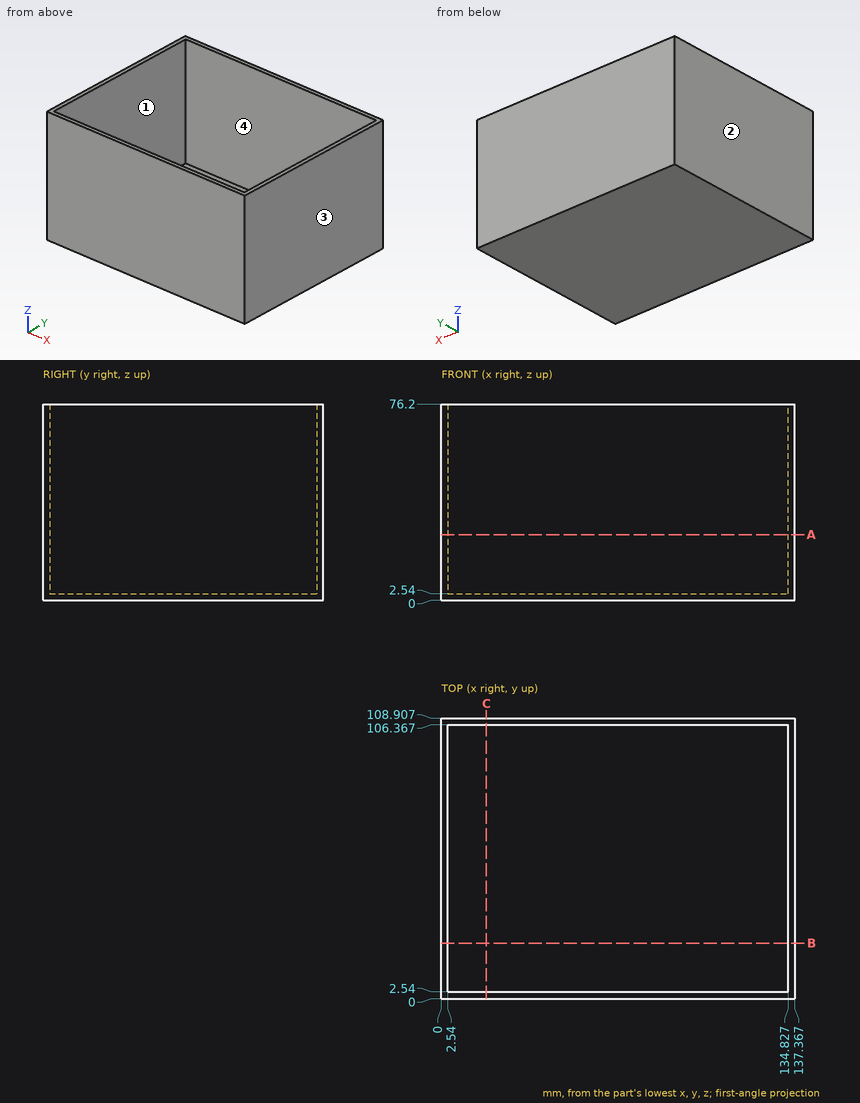
Input: dimensioned drawing with shaded views. Units: mm. Origin: part minimum x, y, z. Coordinates: 2 decimals unless noted, no trailing zeros. Loops run counter-clockwise (first coordinate to the right, second up) from the corner with the lowest first, then second, coordinate; pieces in that order, holes last. Notation, with made-up numbers: (-24.5, 37) - (27.5, 37) arc R15 ccw to (27.5, 66) - close; hole circle Ø9 at (74.25, 23.5). An arc over 180 degrees is marked (long way). One line per question, with ' | ' between items. Start each with the question number.
(1) Cut plane C-C on x = 17.5. Output: boundary loops of the cut face in (y, z).
(2) Ray query, L1, parallel to Y at x = 63.5, z = 60.5; L2, parallel to X at y = 36.5, z = 43; L3, parallel to Z at x = 30, y = 92.5. Return the intervals inside material, ascending. Write a range as from..to.
(3) Cut plane B-B on y = 21.5. Output: boundary loops of the cut face in (x, z).
(4) Draft query along X for the marked faces 1, 2, 3 and 4. Return one class per face: +X half, -X half, draft (parallel to the pull), parting line (faces both ways), or undercut.
(5) First-contact query: pin 1 (2 mm diameter, centred on x = 61.5, y = 82, fed in from +Z). Flat tip, straight axial feed; report the tip coordinate or a pass-through.
(6) Cut plane A-A on z = 25.5. Output: boundary loops of the cut face in (x, y).
Here are the results:
1) outline: (0, 0) - (108.91, 0) - (108.91, 76.2) - (106.37, 76.2) - (106.37, 2.54) - (2.54, 2.54) - (2.54, 76.2) - (0, 76.2) - close
2) L1: 0..2.54, 106.37..108.91 | L2: 0..2.54, 134.83..137.37 | L3: 0..2.54
3) outline: (0, 0) - (137.37, 0) - (137.37, 76.2) - (134.83, 76.2) - (134.83, 2.54) - (2.54, 2.54) - (2.54, 76.2) - (0, 76.2) - close
4) face 1: undercut | face 2: -X half | face 3: +X half | face 4: undercut
5) pin 1: z = 2.54
6) outline: (0, 0) - (137.37, 0) - (137.37, 108.91) - (0, 108.91) - close; hole (2.54, 2.54) - (134.83, 2.54) - (134.83, 106.37) - (2.54, 106.37) - close
